Input: part model. Units: mm. Frame: model coordinates. A direction names the side the tool comes from. Coordinates: 2 decimals unless noted, no trailing zeros. Loops run counter-clockwise (first coordinate to the right, second up) from the corner with the lowest first, then second, coordinate; pieces in that order, holes last. Notation, with made-up numbers: M 5,-30 L 33,-30 A18 ccw 33,-6 Z; hole C 16.5,68 d7. An arc over 180 degrees is marked long. Use a Markdown table: item, result. Add a question column.
1. Draft query along Y for faces 1 (the cylindrical face through (15, -14, 1)), 2 (the flat face through (0, 55, 1)), 3 (the flat face through (-35, -1, 1)). Return one class per face: +Y half, -Y half, draft (parallel to the pull), parting line (faces both ways), or undercut.
2. Section A-A on x = -30. Output: boundary loops of the cut face in (y, z), then the cut area to 3 significant figures.
3. Line query: L1, parallel to Y at x = -30, z = 1.15; L2, parallel to Y at x = 18, z = 1.95; L3, parallel to Y at x = 11.5, z = 1.45. Output: solid intervals per line, ascending. Write a range as [from, to].
4. Section D-D on z = 1.25. Output: boundary loops of the cut face in (x, y), then the cut area to 3 significant figures.
5. Set-up query: faces 4 (the flat face through (35, -1, 1)), 5 (the cylindrical face through (15, 21, 1)). Return all of +Z, -Z, +X, -X, +Y, -Y with unobstructed straight access to the full face (end or side cutting, diameter ignored); none if empty.
6. Section B-B on y = -50. Output: boundary loops of the cut face in (x, z), then the cut area to 3 significant figures.
7. Section C-C on y = 6. Output: boundary loops of the cut face in (x, z), then the cut area to 3 significant figures.
8. Pin query (flat end, axial travel): pin 1 (5 mm diameter, centred on x = -18.5, y = 22.5, fed in from -Z); pin 2 (3.5 mm diameter, centred on x = -9, y = -50, fed in from -Z). Return the tip coordinate at first contact, or that it passes through.
```python
from build123d import *

# Parameters (mm, degrees)
SKIZZE1_W                           = 70
SKIZZE1_H                           = 110
AUFSATZ_LINEAR_AUSTRAGEN1_DEPTH     = 3
DURCHGANGSLOCH_F_R_M41_D            = 4.5
LINEARES_MUSTER1_COUNT              = 2
LINEARES_MUSTER1_PITCH              = 56
LINEARES_MUSTER1_COUNT_DIR2         = 2
LINEARES_MUSTER1_PITCH_DIR2         = 21
F_8_0_8_DURCHMESSER_LANGLOCH4_DEPTH = 3


# Read off the part's stored shape, not the designer's step: Ø8.0 (8) Durchmesser Langloch4
with BuildPart() as part:
    # Skizze1 → Aufsatz-Linear austragen1 (new body)
    with BuildSketch(Plane.XY):
        Rectangle(SKIZZE1_W, SKIZZE1_H)
    extrude(amount=AUFSATZ_LINEAR_AUSTRAGEN1_DEPTH)

    # Durchgangsloch für M41 (through all)
    with Locations(Plane.XY.offset(3)):
        with Locations((-30, -50)):
            durchgangsloch_f_r_m41 = Hole(DURCHGANGSLOCH_F_R_M41_D / 2)

    # Lineares Muster1: Durchgangsloch f_r M41 2 × 2
    with Locations(*[(j * LINEARES_MUSTER1_PITCH_DIR2, i * LINEARES_MUSTER1_PITCH, 0) for i in range(LINEARES_MUSTER1_COUNT) for j in range(LINEARES_MUSTER1_COUNT_DIR2) if (i, j) != (0, 0)]):
        add(durchgangsloch_f_r_m41, mode=Mode.SUBTRACT)

    # Ø8.0 (8) Durchmesser Langloch4 outline → Ø8.0 (8) Durchmesser Langloch4 (cut)
    with BuildSketch(Plane.XY):
        with BuildLine():
            Line((19, -10), (19, 17))
            ThreePointArc((19, 17), (15, 21), (11, 17))
            Line((11, 17), (11, -10))
            ThreePointArc((11, -10), (15, -14), (19, -10))
        make_face()
    extrude(amount=F_8_0_8_DURCHMESSER_LANGLOCH4_DEPTH, mode=Mode.SUBTRACT)


solid = part.part
```
Answers below:
| question | item | result |
|---|---|---|
| 1 | face 1 | undercut |
| 1 | face 2 | +Y half |
| 1 | face 3 | draft |
| 2 | outline | M -55,0 L -52.25,0 L -52.25,3 L -55,3 Z; M -47.75,0 L 3.75,0 L 3.75,3 L -47.75,3 Z; M 8.25,0 L 55,0 L 55,3 L 8.25,3 Z |
| 2 | area | 303 mm² |
| 3 | L1 | y = [-55, -52.25], [-47.75, 3.75], [8.25, 55] |
| 3 | L2 | y = [-55, -12.65], [19.65, 55] |
| 3 | L3 | y = [-55, -11.94], [18.94, 55] |
| 4 | outline | M -35,-55 L 35,-55 L 35,55 L -35,55 Z; hole C -30,-50 d4.5; hole C -30,6 d4.5; hole C -9,-50 d4.5; hole C -9,6 d4.5; hole M 11,-10 A4 ccw 19,-10 L 19,17 A4 ccw 11,17 Z |
| 4 | area | 7,370 mm² |
| 5 | face 4 | +Z, -Z, +X, +Y, -Y |
| 5 | face 5 | +Z, -Z |
| 6 | outline | M -35,0 L -32.25,0 L -32.25,3 L -35,3 Z; M -27.75,0 L -11.25,0 L -11.25,3 L -27.75,3 Z; M -6.75,0 L 35,0 L 35,3 L -6.75,3 Z |
| 6 | area | 183 mm² |
| 7 | outline | M -35,0 L -32.25,0 L -32.25,3 L -35,3 Z; M -27.75,0 L -11.25,0 L -11.25,3 L -27.75,3 Z; M -6.75,0 L 11,0 L 11,3 L -6.75,3 Z; M 19,0 L 35,0 L 35,3 L 19,3 Z |
| 7 | area | 159 mm² |
| 8 | pin 1 | stops at z = 0 |
| 8 | pin 2 | passes through |
